from build123d import *

# Parameters (mm, degrees)
SKETCH1_W            = 148
SKETCH1_H            = 130
SKETCH1_W_2          = 120
SKETCH1_H_2          = 110
BOSS_EXTRUDE2_DEPTH  = 10
SKETCH2_W            = 120
SKETCH2_H            = 24
SKETCH2_W_2          = 118.6
SKETCH2_H_2          = 22.6
SKETCH2_H_3          = 23
SKETCH2_H_4          = 21.6
SKETCH2_H_5          = 5
BOSS_EXTRUDE3_DEPTH  = 1.5
SKETCH3_W            = 120
SKETCH3_H            = 5
BOSS_EXTRUDE4_DEPTH  = 2
SKETCH4_W            = 5
SKETCH4_H            = 110
BOSS_EXTRUDE5_DEPTH  = 3.5
SKETCH5_W            = 5
SKETCH5_H            = 22.6
SKETCH5_H_2          = 21.6
CUT_EXTRUDE1_DEPTH   = 10
SKETCH6_W            = 5
SKETCH6_H            = 0.7
CUT_EXTRUDE2_DEPTH   = 2
SKETCH7_W            = 5
SKETCH7_H            = 24
BOSS_EXTRUDE7_DEPTH  = 3.5
SKETCH8_W            = 0.7
SKETCH8_H            = 22.6
BOSS_EXTRUDE8_DEPTH  = 1.5
SKETCH9_W            = 26
SKETCH9_H            = 0.7
CUT_EXTRUDE3_DEPTH   = 1.5
SKETCH10_W           = 0.7
SKETCH10_H           = 22.6
BOSS_EXTRUDE9_DEPTH  = 1.5
SKETCH11_W           = 5
SKETCH11_H           = 70
BOSS_EXTRUDE10_DEPTH = 3
SKETCH12_W           = 4.519389616
SKETCH12_H           = 130
SKETCH12_W_2         = 4.5
CUT_EXTRUDE4_DEPTH   = 20
SKETCH13_W           = 138.980610384
SKETCH13_H           = 30
SKETCH13_H_2         = 5
CUT_EXTRUDE5_DEPTH   = 20
SKETCH14_W           = 138.980610384
SKETCH14_H           = 3
CUT_EXTRUDE6_DEPTH   = 20
SKETCH15_W           = 4.980610384
SKETCH15_H           = 3
SKETCH15_W_2         = 5
CUT_EXTRUDE7_DEPTH   = 20
SKETCH16_W           = 138.980610384
SKETCH16_H           = 3
CUT_EXTRUDE8_DEPTH   = 200
SKETCH17_W           = 20.6
SKETCH17_H           = 6.4
SKETCH17_H_2         = 5.7
BOSS_EXTRUDE11_DEPTH = 10
BOSS_EXTRUDE12_DEPTH = 20.6
BOSS_EXTRUDE13_DEPTH = 20.6
SKETCH20_W           = 5
SKETCH20_H           = 67
SKETCH20_W_2         = 4.980610384
CUT_EXTRUDE9_DEPTH   = 0.9
SKETCH21_W           = 8.980610384
SKETCH21_H           = 67
BOSS_EXTRUDE14_DEPTH = 1.5


with BuildPart() as part:
    # Sketch1 → Boss-Extrude2 (new body)
    with BuildSketch(Plane(origin=(0, 0, 0), x_dir=(1, 0, 0), z_dir=(0, 1, 0))):
        with Locations((110.217300352, 48.854396258)):
            Rectangle(SKETCH1_W, SKETCH1_H)
        with Locations((110.217300352, 48.854396258)):
            Rectangle(SKETCH1_W_2, SKETCH1_H_2, mode=Mode.SUBTRACT)
    extrude(amount=BOSS_EXTRUDE2_DEPTH)

    # Sketch2 → Boss-Extrude3 (add)
    with BuildSketch(Plane.XZ):
        with Locations((110.217300352, -91.854396258)):
            Rectangle(SKETCH2_W, SKETCH2_H)
        with Locations((110.217300352, -91.854396258)):
            Rectangle(SKETCH2_W_2, SKETCH2_H_2, mode=Mode.SUBTRACT)
        with Locations((110.217300352, -62.854396258)):
            Rectangle(SKETCH2_W, SKETCH2_H)
        with Locations((110.217300352, -62.854396258)):
            Rectangle(SKETCH2_W_2, SKETCH2_H_2, mode=Mode.SUBTRACT)
        with Locations((110.217300352, -33.854396258)):
            Rectangle(SKETCH2_W, SKETCH2_H)
        with Locations((110.217300352, -33.854396258)):
            Rectangle(SKETCH2_W_2, SKETCH2_H_2, mode=Mode.SUBTRACT)
        with Locations((110.217300352, -5.354396258)):
            Rectangle(SKETCH2_W, SKETCH2_H_3)
        with Locations((110.217300352, -5.354396258)):
            Rectangle(SKETCH2_W_2, SKETCH2_H_4, mode=Mode.SUBTRACT)
        with Locations((110.217300352, -19.354396258)):
            Rectangle(SKETCH2_W, SKETCH2_H_5)
        with Locations((110.217300352, -48.354396258)):
            Rectangle(SKETCH2_W, SKETCH2_H_5)
        with Locations((110.217300352, -77.354396258)):
            Rectangle(SKETCH2_W, SKETCH2_H_5)
    extrude(amount=-BOSS_EXTRUDE3_DEPTH)

    # Sketch3 → Boss-Extrude4 (add)
    with BuildSketch(Plane(origin=(0, 1.5, 0), x_dir=(1, 0, 0), z_dir=(0, 1, 0))):
        with Locations((110.217300352, 77.354396258)):
            Rectangle(SKETCH3_W, SKETCH3_H)
        with Locations((110.217300352, 48.354396258)):
            Rectangle(SKETCH3_W, SKETCH3_H)
        with Locations((110.217300352, 19.354396258)):
            Rectangle(SKETCH3_W, SKETCH3_H)
    extrude(amount=BOSS_EXTRUDE4_DEPTH)

    # Sketch4 → Boss-Extrude5 (add)
    with BuildSketch(Plane(origin=(0, 0, 0), x_dir=(-1, 0, 0), z_dir=(0, -1, 0))):
        with Locations((-89.717300352, 48.854396258)):
            Rectangle(SKETCH4_W, SKETCH4_H)
        with Locations((-125.717300352, 48.854396258)):
            Rectangle(SKETCH4_W, SKETCH4_H)
    extrude(amount=-BOSS_EXTRUDE5_DEPTH)

    # Sketch5 → Cut-Extrude1 (cut)
    with BuildSketch(Plane(origin=(0, 0, 0), x_dir=(-1, 0, 0), z_dir=(0, -1, 0))):
        with Locations((-89.717300352, 91.854396258)):
            Rectangle(SKETCH5_W, SKETCH5_H)
        with Locations((-89.717300352, 5.354396258)):
            Rectangle(SKETCH5_W, SKETCH5_H_2)
        with Locations((-89.717300352, 33.854396258)):
            Rectangle(SKETCH5_W, SKETCH5_H)
        with Locations((-89.717300352, 62.854396258)):
            Rectangle(SKETCH5_W, SKETCH5_H)
    extrude(amount=-CUT_EXTRUDE1_DEPTH, mode=Mode.SUBTRACT)

    # Sketch6 → Cut-Extrude2 (cut)
    with BuildSketch(Plane(origin=(0, 1.5, 0), x_dir=(1, 0, 0), z_dir=(0, 1, 0))):
        with Locations((89.717300352, 103.504396258)):
            Rectangle(SKETCH6_W, SKETCH6_H)
        with Locations((89.717300352, 80.204396258)):
            Rectangle(SKETCH6_W, SKETCH6_H)
        with Locations((89.717300352, 74.504396258)):
            Rectangle(SKETCH6_W, SKETCH6_H)
        with Locations((89.717300352, 51.204396258)):
            Rectangle(SKETCH6_W, SKETCH6_H)
        with Locations((89.717300352, 45.504396258)):
            Rectangle(SKETCH6_W, SKETCH6_H)
        with Locations((89.717300352, 22.204396258)):
            Rectangle(SKETCH6_W, SKETCH6_H)
        with Locations((89.717300352, 16.504396258)):
            Rectangle(SKETCH6_W, SKETCH6_H)
        with Locations((89.717300352, -5.795603742)):
            Rectangle(SKETCH6_W, SKETCH6_H)
    extrude(amount=CUT_EXTRUDE2_DEPTH, mode=Mode.SUBTRACT)

    # Sketch7 → Boss-Extrude7 (add)
    with BuildSketch(Plane(origin=(0, 0, 0), x_dir=(-1, 0, 0), z_dir=(0, -1, 0))):
        with Locations((-94.717300352, 91.854396258)):
            Rectangle(SKETCH7_W, SKETCH7_H)
        with Locations((-94.717300352, 62.854396258)):
            Rectangle(SKETCH7_W, SKETCH7_H)
        Polygon((-97.217300352, 16.854396258), (-97.217300352, -6.145603742), (-92.217300352, -6.170565448), (-92.217300352, 16.854396258), align=None)
        with Locations((-94.717300352, 33.854396258)):
            Rectangle(SKETCH7_W, SKETCH7_H)
    extrude(amount=-BOSS_EXTRUDE7_DEPTH)

    # Sketch8 → Boss-Extrude8 (add)
    with BuildSketch(Plane(origin=(0, 0, 0), x_dir=(-1, 0, 0), z_dir=(0, -1, 0))):
        with Locations((-91.867300352, 91.854396258)):
            Rectangle(SKETCH8_W, SKETCH8_H)
        with Locations((-91.867300352, 62.854396258)):
            Rectangle(SKETCH8_W, SKETCH8_H)
        with Locations((-91.867300352, 33.854396258)):
            Rectangle(SKETCH8_W, SKETCH8_H)
    extrude(amount=-BOSS_EXTRUDE8_DEPTH)

    # Sketch9 → Cut-Extrude3 (cut)
    with BuildSketch(Plane(origin=(0, 0, 0), x_dir=(-1, 0, 0), z_dir=(0, -1, 0))):
        Polygon((-50.217300352, 16.854396258), (-92.217300352, 16.854396258), (-92.217300352, 16.154396258), (-50.917300352, 16.154396258), (-50.917300352, -5.445603742), (-92.217300352, -5.445603742), (-92.217300352, -6.145603742), (-50.217300352, -6.145603742), align=None)
        Polygon((-170.217300352, -6.145603742), (-128.217300352, -6.145603742), (-128.217300352, -5.445603742), (-169.517300352, -5.445603742), (-169.517300352, 16.154396258), (-128.217300352, 16.154396258), (-128.217300352, 16.854396258), (-170.217300352, 16.854396258), align=None)
        with Locations((-110.217300352, 16.504396258)):
            Rectangle(SKETCH9_W, SKETCH9_H)
        with Locations((-110.217300352, -5.795603742)):
            Rectangle(SKETCH9_W, SKETCH9_H)
    extrude(amount=-CUT_EXTRUDE3_DEPTH, mode=Mode.SUBTRACT)

    # Sketch10 → Boss-Extrude9 (add)
    with BuildSketch(Plane(origin=(0, 0, 0), x_dir=(-1, 0, 0), z_dir=(0, -1, 0))):
        with Locations((-128.567300352, 91.854396258)):
            Rectangle(SKETCH10_W, SKETCH10_H)
        with Locations((-128.567300352, 62.854396258)):
            Rectangle(SKETCH10_W, SKETCH10_H)
        with Locations((-128.567300352, 33.854396258)):
            Rectangle(SKETCH10_W, SKETCH10_H)
    extrude(amount=-BOSS_EXTRUDE9_DEPTH)

    # Sketch11 → Boss-Extrude10 (add)
    with BuildSketch(Plane(origin=(0, 0, 0), x_dir=(-1, 0, 0), z_dir=(0, -1, 0))):
        with Locations((-43.217300352, 48.854396258)):
            Rectangle(SKETCH11_W, SKETCH11_H)
        with Locations((-177.217300352, 48.854396258)):
            Rectangle(SKETCH11_W, SKETCH11_H)
    extrude(amount=BOSS_EXTRUDE10_DEPTH)

    # Sketch12 → Cut-Extrude4 (cut)
    with BuildSketch(Plane(origin=(0, 10, 0), x_dir=(1, 0, 0), z_dir=(0, 1, 0))):
        with Locations((38.47699516, 48.854396258)):
            Rectangle(SKETCH12_W, SKETCH12_H)
        with Locations((181.967300352, 48.854396258)):
            Rectangle(SKETCH12_W_2, SKETCH12_H)
    extrude(amount=-CUT_EXTRUDE4_DEPTH, mode=Mode.SUBTRACT)

    # Sketch13 → Cut-Extrude5 (cut)
    with BuildSketch(Plane(origin=(0, 0, 0), x_dir=(-1, 0, 0), z_dir=(0, -1, 0))):
        with Locations((-110.22699516, -1.145603742)):
            Rectangle(SKETCH13_W, SKETCH13_H)
        with Locations((-110.22699516, 111.354396258)):
            Rectangle(SKETCH13_W, SKETCH13_H_2)
    extrude(amount=-CUT_EXTRUDE5_DEPTH, mode=Mode.SUBTRACT)

    # Sketch14 → Cut-Extrude6 (cut)
    with BuildSketch(Plane(origin=(0, 0, 0), x_dir=(-1, 0, 0), z_dir=(0, -1, 0))):
        with Locations((-110.22699516, 15.354396258)):
            Rectangle(SKETCH14_W, SKETCH14_H)
    extrude(amount=-CUT_EXTRUDE6_DEPTH, mode=Mode.SUBTRACT)

    # Sketch15 → Cut-Extrude7 (cut)
    with BuildSketch(Plane(origin=(0, -3, 0), x_dir=(-1, 0, 0), z_dir=(0, -1, 0))):
        with Locations((-43.22699516, 15.354396258)):
            Rectangle(SKETCH15_W, SKETCH15_H)
        with Locations((-177.217300352, 15.354396258)):
            Rectangle(SKETCH15_W_2, SKETCH15_H)
    extrude(amount=-CUT_EXTRUDE7_DEPTH, mode=Mode.SUBTRACT)

    # Sketch16 → Cut-Extrude8 (cut)
    with BuildSketch(Plane.XY.offset(-16.854396258)):
        with Locations((110.22699516, 8.5)):
            Rectangle(SKETCH16_W, SKETCH16_H)
    extrude(amount=-CUT_EXTRUDE8_DEPTH, mode=Mode.SUBTRACT)

    # Sketch17 → Boss-Extrude11 (add)
    with BuildSketch(Plane(origin=(0, 0, 0), x_dir=(-1, 0, 0), z_dir=(0, -1, 0))):
        with Locations((-149.217300352, 77.354396258)):
            Rectangle(SKETCH17_W, SKETCH17_H)
        with Locations((-149.217300352, 48.354396258)):
            Rectangle(SKETCH17_W, SKETCH17_H)
        with Locations((-149.217300352, 19.704396258)):
            Rectangle(SKETCH17_W, SKETCH17_H_2)
    extrude(amount=BOSS_EXTRUDE11_DEPTH)

    # Sketch18 → Boss-Extrude12 (add)
    with BuildSketch(Plane.ZY.offset(-138.917300352)):
        with BuildLine():
            Line((-22.554396258, -10), (-16.854396258, -10))
            ThreePointArc((-16.854396258, -10), (-19.704396258, -12.85), (-22.554396258, -10))
        make_face()
        with BuildLine():
            Line((-45.154396258, -10), (-51.554396258, -10))
            ThreePointArc((-51.554396258, -10), (-48.354396258, -13.2), (-45.154396258, -10))
        make_face()
        with BuildLine():
            Line((-74.154396258, -10), (-80.554396258, -10))
            ThreePointArc((-80.554396258, -10), (-77.354396258, -13.2), (-74.154396258, -10))
        make_face()
    extrude(amount=-BOSS_EXTRUDE12_DEPTH)

    # Sketch19 → Boss-Extrude13 (add)
    with BuildSketch(Plane.ZY.offset(-138.917300352)):
        with BuildLine():
            Line((-16.854396258, -10), (-16.854396258, -25))
            ThreePointArc((-16.854396258, -25), (-19.704396258, -27.85), (-22.554396258, -25))
            Line((-22.554396258, -25), (-22.554396258, -10))
            ThreePointArc((-22.554396258, -10), (-19.704396258, -12.85), (-16.854396258, -10))
        make_face()
        with BuildLine():
            Line((-45.154396258, -10), (-45.154396258, -25))
            ThreePointArc((-45.154396258, -25), (-48.354396258, -28.2), (-51.554396258, -25))
            Line((-51.554396258, -25), (-51.554396258, -10))
            Line((-51.554396258, -10), (-45.154396258, -10))
        make_face()
        with BuildLine():
            Line((-74.154396258, -10), (-74.154396258, -25))
            ThreePointArc((-74.154396258, -25), (-77.354396258, -28.2), (-80.554396258, -25))
            Line((-80.554396258, -25), (-80.554396258, -10))
            Line((-80.554396258, -10), (-74.154396258, -10))
        make_face()
    extrude(amount=-BOSS_EXTRUDE13_DEPTH)

    # Sketch20 → Cut-Extrude9 (cut)
    with BuildSketch(Plane(origin=(0, -3, 0), x_dir=(-1, 0, 0), z_dir=(0, -1, 0))):
        with Locations((-177.217300352, 50.354396258)):
            Rectangle(SKETCH20_W, SKETCH20_H)
        with Locations((-43.22699516, 50.354396258)):
            Rectangle(SKETCH20_W_2, SKETCH20_H)
    extrude(amount=-CUT_EXTRUDE9_DEPTH, mode=Mode.SUBTRACT)

    # Sketch21 → Boss-Extrude14 (add)
    with BuildSketch(Plane(origin=(0, -2.1, 0), x_dir=(-1, 0, 0), z_dir=(0, -1, 0))):
        with Locations((-43.22699516, 50.354396258)):
            Rectangle(SKETCH21_W, SKETCH21_H)
        with Locations((-177.22699516, 50.354396258)):
            Rectangle(SKETCH21_W, SKETCH21_H)
    extrude(amount=BOSS_EXTRUDE14_DEPTH)


solid = part.part
Design review of the part built by this model. Coordinates are the model's own, in mm. A direction names the side the tool comes from. Round coordinates to 2 decimals unless told otherwise and drop trailing zeros. Order: outer loops, then holes, each group sorted by start corner. A loop starts at its lowest first (then second) coordinate and runs counter-clockwise, first axis right, second up. Notation, with made-up numbers: M -32.75,63.5 L 1.25,63.5 A30 cw 1.25,97.5 Z; hole C -21,26.5 d6. An arc over 180 degrees is marked long. Answer as CSV lines item,"result". Start each with the question number.
1) Add section A-A (x = 86.5). Give the boundary of the cut face in (y, z), then the cut area to 3 significant figures.
2) For pin 1 Ø3 at (y, z) = (5, -76.5) entering from -X; pin 2 Ø0.8 at (y, z) = (0.5, -61) entering from +X, all flat-tipped, find the tip position at first contact; note any pin that passes through.
3) Add section B-B (y = -18.5). Give the boundary of the cut face in (x, z).
4) Add section C-C (z = -64). Give the number of separate pieces and of enclosed holes in the cut face, then the cut area to 3 significant figures.
5) The part is to be moulded in two halves that separate along Z. For faces 5 (the face through (96, 0, -63)), 6 (the face through (155.5, 1.5, -103.5)), 7 (the face through (43, -2, -83.854)), say which applies: +Z half, -Z half, draft (parallel to the pull), parting line (faces both ways), or undercut.
6) Wall thickness on line 1 along Z through (x, y) = (115.5, 2); line 2 along Z through (x, y) = (153.5, -10); line 3 along Y through (x, z) = (83, -48): over which ranges is each line inside the solid? List them lowest first. Write a range as [from, to].
7) Tool access review of faces 1 (the face through (142.9, 1.5, -22.2)), 2 (the face through (40.737, 3, -62)), 3 (the face through (177, -2, -83.854)), 4 (the face through (149, -12, -74.154)): name each direction out of +Z, -Z, +X, -X, +Y, -Y from which nothing blocks a thin tool from reaching the whole face with its end or side.
Resolved:
1,outline,"M 0,-108.85 L 7,-108.85 L 7,-103.85 L 1.5,-103.85 L 1.5,-103.15 L 0,-103.15 Z; M 0,-80.55 L 1.5,-80.55 L 1.5,-79.85 L 3.5,-79.85 L 3.5,-74.85 L 1.5,-74.85 L 1.5,-74.15 L 0,-74.15 Z; M 0,-51.55 L 1.5,-51.55 L 1.5,-50.85 L 3.5,-50.85 L 3.5,-45.85 L 1.5,-45.85 L 1.5,-45.15 L 0,-45.15 Z; M 0,-22.55 L 1.5,-22.55 L 1.5,-21.85 L 3.5,-21.85 L 3.5,-16.85 L 0,-16.85 Z"
1,area,"93.8 mm^2"
2,pin 1,"x = 40.74"
2,pin 2,"x = 179.72"
3,outline,"M 138.92,-80.55 L 159.52,-80.55 L 159.52,-74.15 L 138.92,-74.15 Z; M 138.92,-51.55 L 159.52,-51.55 L 159.52,-45.15 L 138.92,-45.15 Z; M 138.92,-22.55 L 159.52,-22.55 L 159.52,-16.85 L 138.92,-16.85 Z"
4,separate pieces,"4"
4,enclosed holes,"0"
4,area,"220 mm^2"
5,face 5,"draft"
5,face 6,"undercut"
5,face 7,"-Z half"
6,line 1,"[-108.85, -103.85], [-79.85, -74.85], [-50.85, -45.85], [-21.85, -16.85]"
6,line 2,"[-80.55, -74.15], [-51.55, -45.15], [-22.55, -16.85]"
6,line 3,"[0, 3.5]"
7,face 1,"+Y"
7,face 2,"+Z, -Z, -X, +Y"
7,face 3,"-Z, +X, -X, -Y"
7,face 4,"+Y, -Y"
